Geometry check sheet. Reference: the model listing, model coordinates, mm. Round coordinates to 2 decimals unless told otherwise and drop trailing zeros. Order: outer loops, then holes, each group sorted by start corner. A loop starts at its lowest first (then second) coordinate and runs counter-clockwise, first axis right, second up.
(1) Sectioned sample at B-B (z = 30). Record the boundary of the cut face in (x, y).
(2) Sectioned sample at D-D (y = 9.25). Record the boundary of the cut face in (x, z).
(3) Material ranges on line 1 along Y through (x, z) = (0, 12.75); line 2 along Z through (x, y) = (0, -7.25); line 3 along X through (y, z) = (-7.5, 30), recorded low to high.
(4) Sectioned sample at A-A (x = 0). Record the boundary of the cut face in (y, z), plus the area to 3 significant figures.
(5) Release check for a two-part mould opening along X. For faces 1 (the face through (20, 0, 30)), 2 (the face through (-0.098, 11.744, 49.846)), 3 (the face through (0, 0, 0)), 4 (the face through (-19.1, 12.14, 30.42)) record: +X half, -X half, draft (parallel to the pull), parting line (faces both ways), or undercut.
(6) Go/stop test with a flat-tipped pin: pin 1 (0.9 mm diameter, centred on x = 0, y = -11, fed in from -Z). Record where the tip stops, or that it passes through.
(7) Sectioned sample at C-C (x = -4). Record the boundary of the cut face in (y, z), plus the area to 3 significant figures.
from build123d import *

# Parameters (mm, degrees)
SKETCH1_W           = 40
SKETCH1_H           = 26
SKETCH1_R           = 0.75
BOSS_EXTRUDE1_DEPTH = 60
FILLET1_R           = 3
FILLET2_R           = 3
SKETCH2_R           = 10
CUT_EXTRUDE1_DEPTH  = 27


with BuildPart() as part:
    # Sketch1 → Boss-Extrude1 (new body)
    with BuildSketch(Plane.XY):
        Rectangle(SKETCH1_W, SKETCH1_H)
        with Locations((0, 11)):
            Circle(SKETCH1_R, mode=Mode.SUBTRACT)
        with Locations((0, -11)):
            Circle(SKETCH1_R, mode=Mode.SUBTRACT)
    extrude(amount=BOSS_EXTRUDE1_DEPTH)

    # Fillet1
    fillet1_edges = [part.edges().sort_by_distance(p)[0] for p in [
        (20, 13, 30),
    ]]
    fillet(fillet1_edges, radius=FILLET1_R)

    # Fillet2
    fillet2_edges = [part.edges().sort_by_distance(p)[0] for p in [
        (20, -13, 30),
        (-20, -13, 30),
        (-20, 13, 30),
    ]]
    fillet(fillet2_edges, radius=FILLET2_R)

    # Sketch2 → Cut-Extrude1 (cut, through all)
    with BuildSketch(Plane(origin=(0, 13, 0), x_dir=(1, 0, 0), z_dir=(0, 1, 0))):
        with Locations((0, -30)):
            Circle(SKETCH2_R)
    extrude(amount=-CUT_EXTRUDE1_DEPTH, mode=Mode.SUBTRACT)


solid = part.part
Answer below:
1. outline: (-20, -10) arc R3 ccw to (-17, -13) - (-10, -13) - (-10, 13) - (-17, 13) arc R3 ccw to (-20, 10) - close; (10, -13) - (17, -13) arc R3 ccw to (20, -10) - (20, 10) arc R3 ccw to (17, 13) - (10, 13) - close
2. outline: (-20, 0) - (20, 0) - (20, 60) - (-20, 60) - close; hole circle Ø20 at (0, 30)
3. line 1: y = -13 to -11.75, -10.25 to 10.25, 11.75 to 13
3. line 2: z = 0 to 20, 40 to 60
3. line 3: x = -20 to -10, 10 to 20
4. outline: (-13, 0) - (-11.75, 0) - (-11.75, 20) - (-13, 20) - close; (-13, 40) - (-11.75, 40) - (-11.75, 60) - (-13, 60) - close; (-10.25, 0) - (10.25, 0) - (10.25, 20) - (-10.25, 20) - close; (-10.25, 40) - (10.25, 40) - (10.25, 60) - (-10.25, 60) - close; (11.75, 0) - (13, 0) - (13, 20) - (11.75, 20) - close; (11.75, 40) - (13, 40) - (13, 60) - (11.75, 60) - close
4. area: 920 mm2
5. face 1: +X half
5. face 2: undercut
5. face 3: draft
5. face 4: -X half
6. pin 1: passes through
7. outline: (-13, 0) - (13, 0) - (13, 20.83) - (-13, 20.83) - close; (-13, 39.17) - (13, 39.17) - (13, 60) - (-13, 60) - close
7. area: 1,080 mm2
